CAD build for the part. Positions are in the model's coordinates, mm. A direction names the side the tool comes from. Coordinates: 2 decimals unless noted, no trailing zeros. Loops run counter-clockwise (first coordinate to the right, second up) from the corner with the lowest first, then second, coordinate; pieces in that order, holes last. Notation, with made-up numbers: (-13, -2) -> (-3, -2) arc R5 ccw to (-3, 7) -> close; hole circle Ø6 at (88.5, -5). An arc over 180 degrees is marked (long way). Answer as CSV lines item,"result". Start each with the question number.
from build123d import *

# Parameters (mm, degrees)
F0_R     = 2.5
F0_W     = 5.8
F0_H     = 5.8
F0_R_2   = 1.5
F1_DEPTH = 6


with BuildPart() as f1:
    # F0 (on Front) → F1 (new body)
    with BuildSketch(Plane.XZ):
        with BuildLine():
            Line((-50, 0), (-50, -39))
            Line((-50, -39), (50, -39))
            Line((50, -39), (50, 0))
            Line((50, 0), (64, 0))
            Line((64, 0), (64, 24))
            ThreePointArc((64, 24), (56.58819, 33.659258), (45.339746, 29))
            Line((45.339746, 29), (19.687191, 31.01225))
            ThreePointArc((19.687191, 31.01225), (16.000043, 34.981448), (19.650214, 38.984677))
            Line((19.650214, 38.984677), (54, 42))
            ThreePointArc((54, 42), (59.224972, 41.224972), (64, 38.96663))
            Line((64, 38.96663), (64, 89))
            Line((64, 89), (-64, 89))
            Line((-64, 89), (-64, 38.96663))
            ThreePointArc((-64, 38.96663), (-59.224972, 41.224972), (-54, 42))
            Line((-54, 42), (-19.650214, 38.984677))
            ThreePointArc((-19.650214, 38.984677), (-16.000043, 34.981448), (-19.687191, 31.01225))
            Line((-19.687191, 31.01225), (-45.339746, 29))
            ThreePointArc((-45.339746, 29), (-56.58819, 33.659258), (-64, 24))
            Line((-64, 24), (-64, 0))
            Line((-64, 0), (-50, 0))
        make_face()
        with Locations((-40, -29)):
            Circle(F0_R, mode=Mode.SUBTRACT)
        with Locations((-12.9, -29.9)):
            Rectangle(F0_W, F0_H, mode=Mode.SUBTRACT)
        with Locations((-12.9, -17.9)):
            Rectangle(F0_W, F0_H, mode=Mode.SUBTRACT)
        with Locations((-54, 24)):
            Circle(F0_R_2, mode=Mode.SUBTRACT)
        with Locations((-12.9, -5.9)):
            Rectangle(F0_W, F0_H, mode=Mode.SUBTRACT)
        with Locations((-12.9, 6.1)):
            Rectangle(F0_W, F0_H, mode=Mode.SUBTRACT)
        with Locations((12.9, -29.9)):
            Rectangle(F0_W, F0_H, mode=Mode.SUBTRACT)
        with Locations((12.9, -17.9)):
            Rectangle(F0_W, F0_H, mode=Mode.SUBTRACT)
        with Locations((40, -29)):
            Circle(F0_R, mode=Mode.SUBTRACT)
        with Locations((12.9, -5.9)):
            Rectangle(F0_W, F0_H, mode=Mode.SUBTRACT)
        with Locations((12.9, 6.1)):
            Rectangle(F0_W, F0_H, mode=Mode.SUBTRACT)
        with Locations((54, 24)):
            Circle(F0_R_2, mode=Mode.SUBTRACT)
        with Locations((-40, 79)):
            Circle(F0_R, mode=Mode.SUBTRACT)
        with Locations((40, 79)):
            Circle(F0_R, mode=Mode.SUBTRACT)
    extrude(amount=F1_DEPTH)


solid = f1.part
Item 1: Saw through at B-B (y = -1.05). Count the separate pieces of the cut face and the enclosed holes in it, plus the area to 3 significant figures.
Item 2: Saw through at C-C (x = -39.5). Write the cut outline in (y, z), plus the area to 3 significant figures.
Item 3: Flat gauge pins, fed straight in: pin 1 Ø3 at (y, z) = (-2.5, -6.5) entering from -X; pin 2 Ø1.8 at (x, y) = (-58, -3) entering from -Z. Where does each tip first touch, or does it go through?
Item 4: Saw through at A-A (x = 14). Write the cut outline in (y, z).
Item 5: Saw through at D-D (x = 47.5). Write the cut outline in (y, z), plus the area to 3 significant figures.
Item 6: Two-plate mould, pull along Z, no slides. Class faces 4 (the face through (-54.195, -2.958, 25.487)), 5 (the face through (-64, -3, 64)), 6 (the face through (-10, -3, -6)): pulls with the +Z half, pulls with the -Z half, needs draft (parallel to the pull), parting line crosses it, or undercut.
Item 7: Which spindle directions (+Z, -Z, +X, -X, +Y, -Y) get a long thin tool onto all of the face, cutting with end or side? Do faces 1 (the face through (50, -3, -20)), 2 (the face through (64, -3, 12)), 3 (the face through (-59.3, -3, 41.2)). Say none if no direction does.
Item 8: Wall check: probe 1 along Z at (x, y) = (-11, -4.4); probe 2 along Z at (x, y) = (54, -3.2); probe 3 along X at (y, z) = (-0.6, 8). Give the ranges that are in metal, low to high.
Geometry check:
1,separate pieces,"1"
1,enclosed holes,"14"
1,area,"14,000 mm2"
2,outline,"(-6, -39) -> (0, -39) -> (0, -31.45) -> (-6, -31.45) -> close; (-6, -26.55) -> (0, -26.55) -> (0, 29.46) -> (-6, 29.46) -> close; (-6, 40.73) -> (0, 40.73) -> (0, 76.55) -> (-6, 76.55) -> close; (-6, 81.45) -> (0, 81.45) -> (0, 89) -> (-6, 89) -> close"
2,area,"642 mm2"
3,pin 1,"x = -50"
3,pin 2,"z = 0"
4,outline,"(-6, -39) -> (0, -39) -> (0, -32.8) -> (-6, -32.8) -> close; (-6, -27) -> (0, -27) -> (0, -20.8) -> (-6, -20.8) -> close; (-6, -15) -> (0, -15) -> (0, -8.8) -> (-6, -8.8) -> close; (-6, -3) -> (0, -3) -> (0, 3.2) -> (-6, 3.2) -> close; (-6, 9) -> (0, 9) -> (0, 89) -> (-6, 89) -> close"
5,outline,"(-6, -39) -> (0, -39) -> (0, 31.6) -> (-6, 31.6) -> close; (-6, 41.43) -> (0, 41.43) -> (0, 89) -> (-6, 89) -> close"
5,area,"709 mm2"
6,face 4,"undercut"
6,face 5,"needs draft"
6,face 6,"undercut"
7,face 1,"-Z, +X, +Y, -Y"
7,face 2,"+Z, -Z, +X, +Y, -Y"
7,face 3,"+Y, -Y"
8,probe 1,"-39 to -32.8, -27 to -20.8, -15 to -8.8, -3 to 3.2, 9 to 89"
8,probe 2,"0 to 22.5, 25.5 to 34, 42 to 89"
8,probe 3,"-64 to -15.8, -10 to 10, 15.8 to 64"
